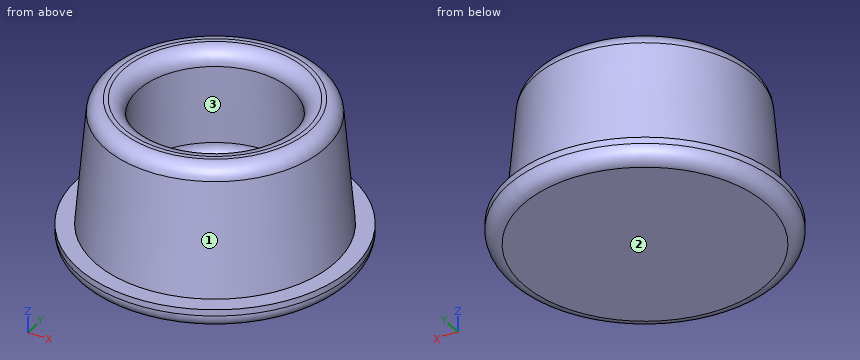
Autodesk Inventor part; units mm, degrees
ref_plane "YZ Plane" through (0, 0, 0) normal (1, 0, 0) x (0, 1, 0)
ref_plane "XZ Plane" through (0, 0, 0) normal (0, 1, 0) x (-1, 0, 0)
ref_plane "XY Plane" through (0, 0, 0) normal (0, 0, 1) x (1, 0, 0)
sketch "Skizze1" plane through (0, 0, 0) normal (0, 1, 0) x (-1, 0, 0)
  line L0 (0, 0) -> (6.5, 0)
  line L1 (6.5, 0) -> (6.5, 1)
  line L2 (6.5, 1) -> (5.7, 1)
  line L3 (5.7, 1) -> (5.1751, 7)
  line L4 (5.1751, 7) -> (0, 7)
  line L5 (0, 7) -> (0, 0)
  line L6 (0, -2.278) -> (0, 8.6565) construction
  dimension "d0" = 6.5
  dimension "d1" = 1
  dimension "d2" = 7
  dimension "d3" = 95
  dimension "d4" = 5.7
revolve "Umdrehung1" add sketch "Skizze1" angle 360 about axis through (0, 0, -2.278) along (0, 0, 1)
fillet "Rundung1" radius 0.7 1 edges at (6.5, 0, 0)
shell "Wandung1" thickness 1.6 removed faces 1 at (1.38, 0.4128, 7)
fillet "Rundung2" radius 0.7 3 edges at (5.1751, 0, 7) (3.569, 0, 7) (4.0414, 0, 1.6)
properties part number "FED ttl plug"
Source: CAD feature listing. Evaluate the final solid. Frame: model axes, mm. Face numbers are marked on the shaded views. Coordinates: 2 decimals unless noted, no trailing zeros. Loops run counter-clockwise (first coordinate to the right, second up) from the corner with the lowest first, then second, coordinate; pieces in that order, holes last. Notation, with made-up numbers: (74, 19.5) - (130, 19.5) arc R31 cw to (130, 43.5) - close; hole circle Ø3 at (-7, 23). An arc over 180 degrees is marked (long way). One line per question, with ' | ' between items.
1) Section C-C, the plane z = 3. Return loops of the section in (x, y).
Report:
outline: circle Ø11.05 at (0, 0); hole circle Ø7.84 at (0, 0)
2) Line query: line 1 along Y through (x, z) = (-1.75, 3.75); line 2 along Y through (x, z) = (2.5, 4.5); line 3 along X through (y, z) = (0.5, 4.5). Output: solid intervals per line, ascending.
Report:
line 1: y = -5.17 to -3.43, 3.43 to 5.17 | line 2: y = -4.78 to -2.85, 2.85 to 4.78 | line 3: x = -5.37 to -3.75, 3.75 to 5.37
3) Section A-A, the plane x = 0. Return loops of the section in (y, z), then the cut area to 3 significant figures.
Report:
outline: (-6.5, 0.7) arc R0.7 ccw to (-5.8, 0) - (5.8, 0) arc R0.7 ccw to (6.5, 0.7) - (6.5, 1) - (5.7, 1) - (5.23, 6.36) arc R0.7 ccw to (4.53, 7) - (4.33, 7) arc R0.7 ccw to (3.64, 6.24) - (3.97, 2.36) arc R0.7 cw to (3.28, 1.6) - (-3.28, 1.6) arc R0.7 cw to (-3.97, 2.36) - (-3.64, 6.24) arc R0.7 ccw to (-4.33, 7) - (-4.53, 7) arc R0.7 ccw to (-5.23, 6.36) - (-5.7, 1) - (-6.5, 1) - close | area: 36.8 mm²
4) Pull-direction query (Y, two-part tool) for the marked faces 1, 2 and 3; classes: released by +Y, released by -Y, zero draft, split by the parting line, or undercut.
Report:
face 1: split by the parting line | face 2: zero draft | face 3: undercut
5) First-contact query: P1, Ø2, axis at y = 2.5, z = 3.5, coming from the -X side; P2, Ø7, axis at x = 1, y = 1, coming from the +Z side; P3, Ø1.5, axis at y = 3.5, z = 4, coming from the -X side. Flat tips, straight axial feed; report the tip coordinate or a pass-through.
Report:
P1: stops at x = -5.29 | P2: stops at z = 7 | P3: stops at x = -4.7
6) Section D-D, the plane z = 3.75. Return loops of the section in (x, y).
Report:
outline: circle Ø10.92 at (0, 0); hole circle Ø7.71 at (0, 0)
